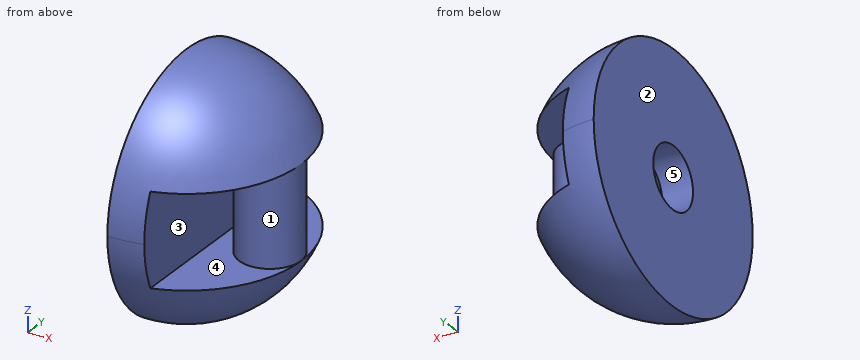
from build123d import *
from build123d.topology import SkipClean

# Parameters (mm, degrees)
SKETCH2_R           = 20
CUT_EXTRUDE1_DEPTH  = 30
SKETCH9_W           = 15
SKETCH9_H           = 41
CUT_EXTRUDE4_DEPTH  = 14.5
SKETCH10_R          = 5
BOSS_EXTRUDE2_DEPTH = 15
SKETCH11_R          = 5
CUT_EXTRUDE5_DEPTH  = 5


with BuildPart() as part:
    # Sketch3 → Revolve1 (revolve)
    with BuildSketch(Plane.XY):
        with BuildLine():
            Line((0, 20), (0, -20))
            ThreePointArc((0, -20), (20, 0), (0, 20))
        make_face()
    revolve(axis=Axis((0, 20, 0), (0, -1, 0)))

    # Sketch2 → Cut-Extrude1 (cut)
    with SkipClean():  # the faces are left unmerged after this step: merging them gives an invalid solid
        with BuildSketch(Plane(origin=(0, 0, 0), x_dir=(0, 0, -1), z_dir=(1, 0, 0))):
            Circle(SKETCH2_R)
        extrude(amount=-CUT_EXTRUDE1_DEPTH, mode=Mode.SUBTRACT)

    # Sketch9 → Cut-Extrude4 (cut)
    with SkipClean():  # the faces are left unmerged after this step: merging them gives an invalid solid
        with BuildSketch(Plane(origin=(20, 0, 0), x_dir=(0, 0, -1), z_dir=(1, 0, 0))):
            Rectangle(SKETCH9_W, SKETCH9_H)
        extrude(amount=-CUT_EXTRUDE4_DEPTH, mode=Mode.SUBTRACT)

    # Sketch10 → Boss-Extrude2 (add)
    with SkipClean():  # the faces are left unmerged after this step: merging them gives an invalid solid
        with BuildSketch(Plane(origin=(0, 0, 7.5), x_dir=(-1, 0, 0), z_dir=(0, 0, -1))):
            with Locations(Location((-13.5, 0, 0), (0, 0, 270))):
                Circle(SKETCH10_R)
        extrude(amount=BOSS_EXTRUDE2_DEPTH)

    # Sketch11 → Cut-Extrude5 (cut)
    with SkipClean():  # the faces are left unmerged after this step: merging them gives an invalid solid
        with BuildSketch(Plane.ZY):
            Circle(SKETCH11_R)
        extrude(amount=-CUT_EXTRUDE5_DEPTH, mode=Mode.SUBTRACT)


solid = part.part
Can you work these out from the model? Positions are in its coordinate system, mm. Face numbers are marked on the shaded views. A direction names the side the tool comes from. Give positions to 0.01 mm unless a question says otherwise; leave off trailing zeros. Write each loop counter-clockwise with the first axis right and the second up, starting at its lowest first coordinate (ties: lowest second). Pieces come first, ordered by that corner, then holes. Notation, with made-up numbers: M 7,64 L 31,64 A13 ccw 31,85 Z; hole C 63.5,35.25 d10. An arc over 180 degrees is marked long. Answer in a Markdown table with one row per item. Add a question column.
Item 1: Imagine slicing it at A-A, the plane y = 0. Write out the boundary of the cut face in (x, z), plus the area to 3 significant figures.
Item 2: On a 3-axis mill with a long thin cutter (end or side, diameter ignored), from which of +Z, -Z, +X, -X, +Y, -Y can I reach the whole of each face in a straight line? I mean the marked faces 3, 4 and 5. Say none if no direction works.
Item 3: Imagine slicing it at D-D, the plane y = 5.5. Write out the boundary of the cut face in (x, z).
Item 4: For pin 1 Ø6 at (x, y) = (7, -6) entering from +Z; pin 2 Ø3 at (x, y) = (10.5, -8) entering from +Z; pin 3 Ø10.5 at (x, y) = (13.5, 4.5) entering from +Z, each with a flat end and sliding along its axis, tell me the tip position at first contact or that it passes through.
Item 5: Imagine slicing it at C-C, the plane x = 10.5. Write out the boundary of the cut face in (y, z), plus the area to 3 significant figures.
Item 6: We'd pull the mould along Z, two halves only. Please class the marked faces 1 and 2: released by +Z, released by -Z, zero draft, split by the parting line, or undercut.
Item 7: Imagine slicing it at B-B, the plane z = 1.5. Write out the boundary of the cut face in (x, y).
Item 8: Please list where these lines run through material, in increasing order: L1, parallel to X at y = -10.5, z = 2; L2, parallel to Y at x = 2.5, z = 0; L3, parallel to Z at x = 2.75, y = 0.5.
Evaluation:
| question | item | result |
|---|---|---|
| 1 | outline | M 0,-20 A20 ccw 18.54,-7.5 L 18.5,-7.5 L 18.5,7.5 L 18.54,7.5 A20 ccw 0,20 L 0,5 L 5,5 L 5,-5 L 0,-5 Z; hole M 5.5,-7.5 L 8.5,-7.5 L 8.5,7.5 L 5.5,7.5 Z |
| 1 | area | 518 mm² |
| 2 | face 3 | +Y, -Y |
| 2 | face 4 | none |
| 2 | face 5 | -X |
| 3 | outline | M 0,-19.23 A19.23 ccw 17.71,-7.5 L 5.5,-7.5 L 5.5,7.5 L 17.71,7.5 A19.23 ccw 0,19.23 Z |
| 4 | pin 1 | stops at z = 19.01 |
| 4 | pin 2 | stops at z = 16.22 |
| 4 | pin 3 | stops at z = 17.87 |
| 5 | outline | M -15.28,-7.5 A17.02 ccw 15.28,-7.5 L 4,-7.5 L 4,7.5 L 15.28,7.5 A17.02 ccw -15.28,7.5 L -4,7.5 L -4,-7.5 Z |
| 5 | area | 537 mm² |
| 6 | face 1 | undercut |
| 6 | face 2 | zero draft |
| 7 | outline | M 0,-19.94 A19.94 ccw 5.5,-19.17 L 5.5,19.17 A19.94 ccw 0,19.94 L 0,4.77 L 5,4.77 L 5,-4.77 L 0,-4.77 Z; C 13.5,0 d10 |
| 8 | L1 | x = 0 to 5.5 |
| 8 | L2 | y = -19.84 to -5, 5 to 19.84 |
| 8 | L3 | z = -19.8 to -4.97, 4.97 to 19.8 |
